from build123d import *

# Parameters (mm, degrees)
SKETCH3_R           = 7.5
BOSS_EXTRUDE1_DEPTH = 27.5
CHAMFER1_SIZE       = 0.75
FILLET2_R           = 0.5625


with BuildPart() as part:
    # Sketch3 → Boss-Extrude1 (new, symmetric)
    with BuildSketch(Plane.XY):
        Circle(SKETCH3_R)
    extrude(amount=BOSS_EXTRUDE1_DEPTH, both=True)

    # Chamfer1
    chamfer1_edges = [part.edges().sort_by_distance(p)[0] for p in [
        (-7.5, 0, -27.5),
        (-7.5, 0, 27.5),
    ]]
    chamfer(chamfer1_edges, length=CHAMFER1_SIZE)

    # Fillet2
    fillet2_edges = [part.edges().sort_by_distance(p)[0] for p in [
        (-7.5, 0, -26.75),
        (-7.5, 0, 26.75),
    ]]
    fillet(fillet2_edges, radius=FILLET2_R)


solid = part.part
Work out the finished part from the listing and answer in its coordinate system (mm). Give positions to 0.01 mm unless a question says otherwise; leave off trailing zeros. Loops run counter-clockwise (first coordinate to the right, second up) from the corner with the lowest first, then second, coordinate; pieces in that order, holes last. Notation, with made-up numbers: (-32, 16) - (0, 16) arc R19 cw to (0, 39) - close; hole circle Ø8 at (45, 66.25). An arc over 180 degrees is marked (long way). Answer in a Markdown table with one row per item. Add a question column.
Q1. Each of these flat-tipped pins is pushed along its axis until it touches: P1, Ø2, axis at y = 1, z = -3.5, coming from the +X side; P2, Ø2, axis at y = 2.5, z = 11.5, coming from the -X side; P3, Ø3, axis at x = 5, z = -2, coming from the +Y side. Where does it stop, or does it pass through?
Q2. The part is cut by section A-A (z = -1.5). Determine the outline of the cut face in (x, y).
Q3. Consider line 1 along X through (y, z) = (-0.25, -13); line 2 along Z through (x, y) = (6.75, -2); line 3 along Y through (x, z) = (3, 5). Determine where each line is inside the solid, lowest interval first.
Solution:
| question | item | result |
|---|---|---|
| 1 | P1 | stops at x = 7.5 |
| 1 | P2 | stops at x = -7.35 |
| 1 | P3 | stops at y = 6.63 |
| 2 | outline | circle Ø15 at (0, 0) |
| 3 | line 1 | x = -7.5 to 7.5 |
| 3 | line 2 | z = -27.21 to 27.21 |
| 3 | line 3 | y = -6.87 to 6.87 |
